```python
from build123d import *

# Parameters (mm, degrees)
SKETCH1_R                       = 42
BOSS_EXTRUDE1_DEPTH             = 3
SKETCH2_W                       = 70
SKETCH2_H                       = 25
BOSS_EXTRUDE2_DEPTH             = 3
SKETCH3_R                       = 34.5
CUT_EXTRUDE1_DEPTH              = 1
CUT_EXTRUDE1_DEPTH_BACK         = 4
CUT_EXTRUDE2_DEPTH              = 1
CUT_EXTRUDE2_DEPTH_BACK         = 4
CUT_EXTRUDE3_START              = -4
SKETCH5_R                       = 2.25
CUT_EXTRUDE3_DEPTH              = 5
CIRPATTERN1_COUNT               = 12
SKETCH6_R                       = 122.183782822
SKETCH6_R_2                     = 65
CUT_EXTRUDE4_DEPTH              = 4
CUT_EXTRUDE4_DEPTH_BACK         = 1
CUT_EXTRUDE5_START              = -4
SKETCH7_R                       = 2.25
CUT_EXTRUDE5_DEPTH              = 5
CIRPATTERN2_COUNT               = 2
CIRPATTERN2_ANGLE               = 8
CIRPATTERN2_THE_OTHER_WAY_COUNT = 2
CIRPATTERN2_THE_OTHER_WAY_ANGLE = 8


with BuildPart() as part:
    # Sketch1 → Boss-Extrude1 (new body)
    with BuildSketch(Plane(origin=(0, 0, 0), x_dir=(1, 0, 0), z_dir=(0, 1, 0))):
        Circle(SKETCH1_R)
    extrude(amount=BOSS_EXTRUDE1_DEPTH)

    # Sketch2 → Boss-Extrude2 (add)
    with BuildSketch(Plane(origin=(0, 0, 0), x_dir=(1, 0, 0), z_dir=(0, 1, 0))):
        with Locations((35, 0)):
            Rectangle(SKETCH2_W, SKETCH2_H)
    extrude(amount=BOSS_EXTRUDE2_DEPTH)

    # Sketch3 → Cut-Extrude1 (cut, two sides)
    with BuildSketch(Plane(origin=(0, 3, 0), x_dir=(1, 0, 0), z_dir=(0, 1, 0))) as cut_extrude1_sk:
        Circle(SKETCH3_R)
    extrude(amount=CUT_EXTRUDE1_DEPTH, mode=Mode.SUBTRACT)
    extrude(cut_extrude1_sk.sketch, amount=-CUT_EXTRUDE1_DEPTH_BACK, mode=Mode.SUBTRACT)

    # Sketch4 → Cut-Extrude2 (cut, two sides)
    with BuildSketch(Plane(origin=(0, 3, 0), x_dir=(1, 0, 0), z_dir=(0, 1, 0))) as cut_extrude2_sk:
        with BuildLine():
            Line((0, 0), (40.099953579, -12.489744711))
            ThreePointArc((40.099953579, -12.489744711), (-26.884607378, -32.267907991), (-19.52336592, 37.186532282))
            Line((-19.52336592, 37.186532282), (0, 0))
        make_face()
    extrude(amount=CUT_EXTRUDE2_DEPTH, mode=Mode.SUBTRACT)
    extrude(cut_extrude2_sk.sketch, amount=-CUT_EXTRUDE2_DEPTH_BACK, mode=Mode.SUBTRACT)

    # Sketch5 → Cut-Extrude3 (cut)
    with BuildSketch(Plane(origin=(0, 3, 0), x_dir=(1, 0, 0), z_dir=(0, 1, 0)).offset(CUT_EXTRUDE3_START)):
        with Locations((-12.996765446, 35.70831959)):
            Circle(SKETCH5_R)
    cut_extrude3 = extrude(amount=CUT_EXTRUDE3_DEPTH, mode=Mode.SUBTRACT)

    # CirPattern1: Cut-Extrude3 ×12 about axis
    cirpattern1_axis = Axis((0, 0, 0), (0, -1, 0))
    for i in range(1, CIRPATTERN1_COUNT):
        add(cut_extrude3.rotate(cirpattern1_axis, i * 360 / CIRPATTERN1_COUNT), mode=Mode.SUBTRACT)

    # Sketch6 → Cut-Extrude4 (cut, two sides)
    with BuildSketch(Plane(origin=(0, 0, 0), x_dir=(1, 0, 0), z_dir=(0, 1, 0))) as cut_extrude4_sk:
        Circle(SKETCH6_R)
        Circle(SKETCH6_R_2, mode=Mode.SUBTRACT)
    extrude(amount=CUT_EXTRUDE4_DEPTH, mode=Mode.SUBTRACT)
    extrude(cut_extrude4_sk.sketch, amount=-CUT_EXTRUDE4_DEPTH_BACK, mode=Mode.SUBTRACT)

    # Sketch7 → Cut-Extrude5 (cut)
    with BuildSketch(Plane(origin=(0, 3, 0), x_dir=(1, 0, 0), z_dir=(0, 1, 0)).offset(CUT_EXTRUDE5_START)):
        with Locations((60, 0)):
            Circle(SKETCH7_R)
    cut_extrude5 = extrude(amount=CUT_EXTRUDE5_DEPTH, mode=Mode.SUBTRACT)

    # CirPattern2: Cut-Extrude5 ×2 about axis
    cirpattern2_axis = Axis((0, 3, 0), (0, 1, 0))
    for i in range(1, CIRPATTERN2_COUNT):
        add(cut_extrude5.rotate(cirpattern2_axis, i * CIRPATTERN2_ANGLE / (CIRPATTERN2_COUNT - 1)), mode=Mode.SUBTRACT)

    # CirPattern2 the other way: Cut-Extrude5 ×2 about axis
    cirpattern2_the_other_way_axis = Axis((0, 3, 0), (0, -1, 0))
    for i in range(1, CIRPATTERN2_THE_OTHER_WAY_COUNT):
        add(cut_extrude5.rotate(cirpattern2_the_other_way_axis, i * CIRPATTERN2_THE_OTHER_WAY_ANGLE / (CIRPATTERN2_THE_OTHER_WAY_COUNT - 1)), mode=Mode.SUBTRACT)


solid = part.part
```
Work out the finished part from the listing and answer in its coordinate system (mm). Give positions to 0.01 mm unless a question says otherwise; leave off trailing zeros. Write each loop counter-clockwise with the first axis right and the second up, starting at its lowest first coordinate (ties: lowest second). Pieces come first, ordered by that corner, then holes.
(1) The part is cut by section C-C on y = 0.95. Count the separate pieces of the cut face and the enclosed holes in it, plus the area to 3 significant figures.
Final values:
separate pieces: 1
enclosed holes: 8
area: 1,130 mm2
(2) The part is cut by section A-A on z = 0. Write down the section's boundary in (x, y).
Final values:
outline: (34.5, 0) - (57.75, 0) - (57.75, 3) - (34.5, 3) - close; (62.25, 0) - (65, 0) - (65, 3) - (62.25, 3) - close
(3) The part is cut by section B-B on x = 60. Write down the section's boundary in (y, z), plus the area to 3 significant figures.
Final values:
outline: (0, -12.5) - (3, -12.5) - (3, -10.52) - (0, -10.52) - close; (0, -6.18) - (3, -6.18) - (3, -2.25) - (0, -2.25) - close; (0, 2.25) - (3, 2.25) - (3, 6.18) - (0, 6.18) - close; (0, 10.52) - (3, 10.52) - (3, 12.5) - (0, 12.5) - close
area: 35.4 mm2
(4) The part is cut by section D-D on z = -28.5. Write down the section's boundary in (x, y), plus the area to 3 significant figures.
Final values:
outline: (19.44, 0) - (22.26, 0) - (22.26, 3) - (19.44, 3) - close; (26.59, 0) - (30.85, 0) - (30.85, 3) - (26.59, 3) - close
area: 21.2 mm2
(5) Straight lines are drawn through the part: line 1 (X direction, y = 2.9, z = -37); line 2 (Z direction, x = 37, y = 0.95); line 3 (Z direction, x = 60, y = 2.35). For each, find the intervals that lie inside material, in ascending order.
Final values:
line 1: x = -19.43 to -14.84, -11.15 to 4.39, 8.81 to 19.87
line 2: z = -19.87 to -14.84, -11.15 to 4.39, 8.81 to 11.52
line 3: z = -12.5 to -10.52, -6.18 to -2.25, 2.25 to 6.18, 10.52 to 12.5
(6) Flat-ended cylindrical pins translate along their axes: pin 1 Ø4 at (x, z) = (60, 0) entering from -Y; pin 2 Ø1.5 at (x, y) = (-4.5, 2) entering from +Z; pin 3 Ø6 at (x, z) = (-13, -35.71) entering from -Y. Find the tip coordinate at first contact, or state that the pin passes through.
Final values:
pin 1: passes through
pin 2: stops at z = -34.1
pin 3: stops at y = 0
(7) The mould has two halves that part along X. Classify faces 1 (the cylindrical face through (65, 1, 0)), 2 (the flat face through (36.47, 1.52, 11.36)), 3 (the cylindrical face through (61.594, 1.479, -7.786)), 4 (the flat face through (52, 1, -12.5)): pulls with the +X half, pulls with the -X half, needs draft (parallel to the pull), parting line crosses it, or undercut.
Final values:
face 1: pulls with the +X half
face 2: pulls with the -X half
face 3: undercut
face 4: needs draft
